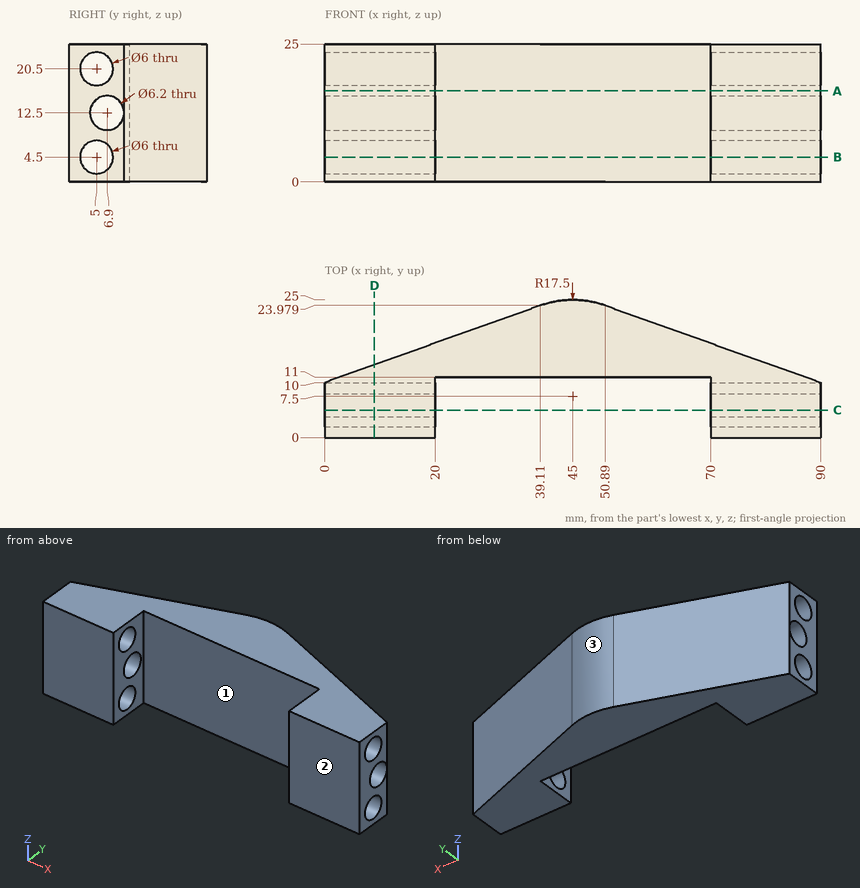
Here's the drawing with two shaded views (mm, measured from the low corner). I have some questions. Round coordinates to 2 decimals unless told otherwise and drop trailing zeros. Order: outer loops, then holes, each group sorted by start corner. A loop starts at its lowest first (then second) coordinate and runs counter-clockwise, first axis right, second up. Notation, with made-up numbers: (0, 88) -> (4, 88) arc R36 ccw to (4, 122) -> close; hole circle Ø7 at (5, 26.25). An arc over 180 degrees is marked (long way). Return JSON: item names as keys, results as strings.
Q1. If we section it at B-B on z = 4.5: List the corners of the cut face in (x, y) for me.
Filled sheet:
{"outline": "(0, 0) -> (20, 0) -> (20, 2) -> (0, 2) -> close; (0, 8) -> (20, 8) -> (20, 11) -> (70, 11) -> (70, 8) -> (90, 8) -> (90, 10) -> (50.89, 23.98) arc R17.5 ccw to (39.11, 23.98) -> (0, 10) -> close; (70, 0) -> (90, 0) -> (90, 2) -> (70, 2) -> close"}
Q2. If we section it at D-D on x = 9: List the corners of the cut face in (y, z) for me.
Filled sheet:
{"outline": "(0, 0) -> (13.22, 0) -> (13.22, 25) -> (0, 25) -> close; hole circle Ø6 at (5, 4.5); hole circle Ø6 at (5, 20.5); hole circle Ø6.2 at (6.9, 12.5)"}
Q3. I need wall thicknesses on line 1 along X through (y, z) = (2, 13.25); line 2 along Z through (x, y) = (12.25, 6.9); line 3 along Z through (x, y) = (6, 5). Which ranges of each line are inside material? Lowest first, please. Write a range as from..to.
Filled sheet:
{"line 1": "x = 0..20, 70..90", "line 2": "z = 0..2.18, 6.82..9.4, 15.6..18.18, 22.82..25", "line 3": "z = 0..1.5, 7.5..10.05, 14.95..17.5, 23.5..25"}
Q4. For pin 1 Ø6 at (x, z) = (68, 16) entering from +Y; pin 2 Ø6 at (x, z) = (57.5, 10.5) entering from +Y; pin 3 Ø5 at (x, z) = (39.5, 4.5) entering from +Y, each with a flat end and sliding along its axis, tell me the tip position at first contact or that it passes through.
Filled sheet:
{"pin 1": "stops at y = 18.94", "pin 2": "stops at y = 22.69", "pin 3": "stops at y = 24.74"}
Q5. If we section it at A-A on z = 16.5: List the corners of the cut face in (x, y) for me, plus the area to 3 significant figures.
Filled sheet:
{"outline": "(0, 0) -> (20, 0) -> (20, 11) -> (70, 11) -> (70, 0) -> (90, 0) -> (90, 10) -> (50.89, 23.98) arc R17.5 ccw to (39.11, 23.98) -> (0, 10) -> close", "area": "1,070 mm^2"}
Q6. If we mould it in two halves opening along X, with no side actions, what happens to the marked faces 1, 2 and 3? For each: released by +X, released by -X, zero draft, split by the parting line, or undercut.
Filled sheet:
{"face 1": "undercut", "face 2": "zero draft", "face 3": "split by the parting line"}
Q7. If we section it at C-C on y = 5: Give the number of separate pieces and of enclosed holes in the cut face, plus the area to 3 significant figures.
Filled sheet:
{"separate pieces": "8", "enclosed holes": "0", "area": "324 mm^2"}
